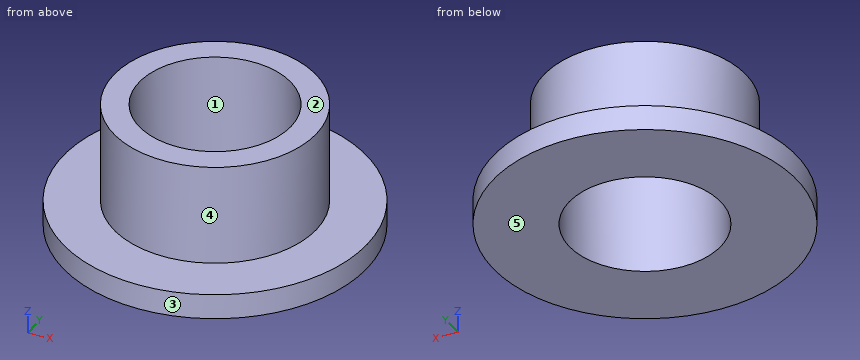
Autodesk Inventor part; units mm, degrees
ref_plane "YZ Plane" through (0, 0, 0) normal (1, 0, 0) x (0, 1, 0)
ref_plane "XZ Plane" through (0, 0, 0) normal (0, 1, 0) x (-1, 0, 0)
ref_plane "XY Plane" through (0, 0, 0) normal (0, 0, 1) x (1, 0, 0)
sketch "スケッチ1" plane through (0, 0, 0) normal (0, 0, 1) x (1, 0, 0)
  circle A0 centre (0, 0) radius 6
  dimension "d0" = 12
extrude "押し出し1" add sketch "スケッチ1" along normal blind 1
sketch "スケッチ2" plane through (0, 0, 1) normal (0, 0, 1) x (1, 0, 0)
  circle A0 centre (0, 0) radius 4
  dimension "d3" = 8
extrude "押し出し2" add sketch "スケッチ2" along normal blind 4
sketch "スケッチ3" plane through (0, 0, 5) normal (0, 0, 1) x (1, 0, 0)
  circle A0 centre (0, 0) radius 3
  dimension "d6" = 6
extrude "押し出し3" cut sketch "スケッチ3" against normal through all
properties part number "oiles_bush6" material "ABS プラスチック"
CAD build for the part. Positions are in the model's coordinates, mm. Face numbers are marked on the shaded views. A direction names the side the tool comes from. Give positions to 0.01 mm unless a question says otherwise; leave off trailing zeros. Order: outer loops, then holes, each group sorted by start corner. A loop starts at its lowest first (then second) coordinate and runs counter-clockwise, first axis right, second up. Notation, with made-up numbers: (-4, 41.25) -> (43, 41.25) arc R6 ccw to (43, 47.25) -> close; hole circle Ø4 at (72.5, -31.75). An arc over 180 degrees is marked (long way). Return JSON: item names as keys, results as strings.
Q1. Mould opens along X. For the marked faces 1, 2 and 3 say: pulls with the +X half, pulls with the -X half, needs draft (parallel to the pull), parting line crosses it, or undercut.
Working result:
{"face 1": "undercut", "face 2": "needs draft", "face 3": "parting line crosses it"}
Q2. Saw through at D-D (y = -3.5). Write the cut outline in (x, z).
Working result:
{"outline": "(-4.87, 0) -> (4.87, 0) -> (4.87, 1) -> (1.94, 1) -> (1.94, 5) -> (-1.94, 5) -> (-1.94, 1) -> (-4.87, 1) -> close"}
Q3. Which spindle directions (+Z, -Z, +X, -X, +Y, -Y) get a long thin tool onto all of the face, cutting with end or side? Do the marked faces 4 and 5. Say none if no direction does.
Working result:
{"face 4": "+Z", "face 5": "-Z, +X, -X, +Y, -Y"}
Q4. Saw through at A-A (y = 0). Write the cut outline in (x, z), then the cut area to 3 significant figures.
Working result:
{"outline": "(-6, 0) -> (-3, 0) -> (-3, 5) -> (-4, 5) -> (-4, 1) -> (-6, 1) -> close; (3, 0) -> (6, 0) -> (6, 1) -> (4, 1) -> (4, 5) -> (3, 5) -> close", "area": "14.0 mm²"}
Q5. Saw through at C-C (z = 0.45). Write the cut outline in (x, y).
Working result:
{"outline": "circle Ø12 at (0, 0); hole circle Ø6 at (0, 0)"}
Q6. Drill centre lines: line 1 (Y direction, x = 0, z = 4.6); line 2 (Z direction, x = 3.75, y = -4.5); line 3 (X direction, y = -1.75, z = 3.1). Where is each one in solid material? Low to high.
Working result:
{"line 1": "-4 to -3, 3 to 4", "line 2": "0 to 1", "line 3": "-3.6 to -2.44, 2.44 to 3.6"}
Q7. Flat gauge pins, fed straight in: pin 1 (1 mm diameter, centred on y = -1, z = 3.5, fed in from -X); pin 2 (1.5 mm diameter, centred on x = -3.5, y = -4, fed in from +Z); pin 3 (2 mm diameter, centred on y = -2, z = 2.5, fed in from -X). Where does each tip first touch, or does it go through?
Working result:
{"pin 1": "x = -3.97", "pin 2": "z = 1", "pin 3": "x = -3.87"}
